Could you check a few things on this model? Use its own coordinates, in mm. A direction names the side the tool comes from. Coordinates: 2 decimals unless noted, no trailing zeros. Write each loop counter-clockwise with the first axis right and the second up, starting at its lowest first coordinate (ties: lowest second). Pieces come first, ordered by that corner, then holes.
```python
from build123d import *

# Parameters (mm, degrees)
ESQUISSE1_W             = 34
ESQUISSE1_H             = 21
BOSS_EXTRU_1_DEPTH      = 3
ESQUISSE2_W             = 30
ESQUISSE2_H             = 12
BOSS_EXTRU_2_DEPTH      = 1.5
ESQUISSE3_R             = 1
ESQUISSE3_R_2           = 1.25
ENL_V_MAT_EXTRU_1_DEPTH = 5


with BuildPart() as part:
    # Esquisse1 → Boss.-Extru.1 (new body)
    with BuildSketch(Plane(origin=(0, 0, 0), x_dir=(1, 0, 0), z_dir=(0, 1, 0))):
        with Locations((17, 10.5)):
            Rectangle(ESQUISSE1_W, ESQUISSE1_H)
    extrude(amount=BOSS_EXTRU_1_DEPTH)

    # Esquisse2 → Boss.-Extru.2 (add)
    with BuildSketch(Plane(origin=(0, 3, 0), x_dir=(1, 0, 0), z_dir=(0, 1, 0))):
        with Locations((17, 11)):
            Rectangle(ESQUISSE2_W, ESQUISSE2_H)
    extrude(amount=BOSS_EXTRU_2_DEPTH)

    # Esquisse3 → Enlèv. mat.-Extru.1 (cut)
    with BuildSketch(Plane(origin=(0, 3, 0), x_dir=(1, 0, 0), z_dir=(0, 1, 0))):
        with Locations(Location((11, 2, 0), (0, 0, 270))):
            Circle(ESQUISSE3_R)
        with Locations(Location((13.5, 2, 0), (0, 0, 270))):
            Circle(ESQUISSE3_R)
        with Locations(Location((16, 2, 0), (0, 0, 270))):
            Circle(ESQUISSE3_R)
        with Locations(Location((18.5, 2, 0), (0, 0, 270))):
            Circle(ESQUISSE3_R)
        with Locations(Location((21, 2, 0), (0, 0, 270))):
            Circle(ESQUISSE3_R)
        with Locations(Location((23.5, 2, 0), (0, 0, 270))):
            Circle(ESQUISSE3_R)
        with Locations(Location((2, 2, 0), (0, 0, 270))):
            Circle(ESQUISSE3_R_2)
        with Locations(Location((2, 19, 0), (0, 0, 270))):
            Circle(ESQUISSE3_R_2)
        with Locations(Location((32, 19, 0), (0, 0, 270))):
            Circle(ESQUISSE3_R_2)
        with Locations(Location((32, 2, 0), (0, 0, 270))):
            Circle(ESQUISSE3_R_2)
    extrude(amount=-ENL_V_MAT_EXTRU_1_DEPTH, mode=Mode.SUBTRACT)


solid = part.part
```
1. For pin 1 (2 mm diameter, centred on x = 32, z = -2, fed in from +Y), with a flat end and sliding along its axis, tell me the tip position at first contact or that it passes through.
Verdict:
pin 1: passes through
2. I want a section at D-D on x = 31.5. Please give me the cut outline in (y, z), plus the area to 3 significant figures.
Verdict:
outline: (0, -21) - (3, -21) - (3, -20.15) - (0, -20.15) - close; (0, -17.85) - (3, -17.85) - (3, -17) - (4.5, -17) - (4.5, -5) - (3, -5) - (3, -3.15) - (0, -3.15) - close; (0, -0.85) - (3, -0.85) - (3, 0) - (0, 0) - close
area: 67.3 mm2
3. I want a section at B-B on x = 13.5. Please give me the cut outline in (y, z), plus the area to 3 significant figures.
Verdict:
outline: (0, -21) - (3, -21) - (3, -17) - (4.5, -17) - (4.5, -5) - (3, -5) - (3, -3) - (0, -3) - close; (0, -1) - (3, -1) - (3, 0) - (0, 0) - close
area: 75.0 mm2
4. I want a section at C-C on y = 0.8. Give the number of separate pieces and of enclosed holes in the cut face, plus the area to 3 significant figures.
Verdict:
separate pieces: 1
enclosed holes: 10
area: 676 mm2
5. Please list where these lines run through material, in increasing order: line 1 along X through (y, z) = (0.65, -19); line 2 along Y through (x, z) = (6.5, -17.5); line 3 along Z through (x, y) = (28, 3.65).
Verdict:
line 1: x = 0 to 0.75, 3.25 to 30.75, 33.25 to 34
line 2: y = 0 to 3
line 3: z = -17 to -5
6. I want a section at A-A on z = -19. Please give me the cut outline in (x, y), plus the area to 3 significant figures.
Verdict:
outline: (0, 0) - (0.75, 0) - (0.75, 3) - (0, 3) - close; (3.25, 0) - (30.75, 0) - (30.75, 3) - (3.25, 3) - close; (33.25, 0) - (34, 0) - (34, 3) - (33.25, 3) - close
area: 87.0 mm2
7. If we mould it in two halves opening along Y, with no side actions, what happens to faces 1 (the face through (17, 4.5, -11)), 2 (the face through (22.524, 1.521, -2.217)), 3 (the face through (17, 0, -11))? For each: pulls with the +Y half, pulls with the -Y half, needs draft (parallel to the pull), parting line crosses it, or undercut.
Verdict:
face 1: pulls with the +Y half
face 2: needs draft
face 3: pulls with the -Y half
8. On a 3-axis mill with a long thin cutter (end or side, diameter ignored), from which of +Z, -Z, +X, -X, +Y, -Y can I reach the whole of each face in a straight line? I mean faces 4 (the face through (17, 4, -5)), 5 (the face through (32, 4, -11)), 6 (the face through (17, 4, -17)). Say none if no direction works.
Verdict:
face 4: +Z, +X, -X, +Y
face 5: +Z, -Z, +X, +Y
face 6: -Z, +X, -X, +Y
